Autodesk Inventor part; units mm, degrees
ref_plane "Work Plane2" through (-342.433406, -360.707407, -533) normal (0, 0, -1) x (0, 1, 0)
ref_plane "YZ Plane" through (0, 0, 0) normal (1, 0, 0) x (0, 1, 0)
ref_plane "XZ Plane" through (0, 0, 0) normal (0, 1, 0) x (-1, 0, 0)
ref_plane "Work Plane1" through (0, 0, 0) normal (0, 0, 1) x (1, 0, 0)
sketch "Sketch1" plane through (0, 0, 0) normal (0, 0, 1) x (1, 0, 0)
  arc A0 (173.074137, -21.982113) -> (67.5, 160.877656) centre (67.5, 38.971143) ccw
  line L0 (67.5, 160.877656) -> (23, 160.877656)
  line L1 (150.824137, -60.520244) -> (173.074137, -21.982113)
  line L2 (23, 162.377656) -> (67.5, 162.377656)
  arc A1 (174.373175, -22.732113) -> (67.5, 162.377656) centre (67.5, 38.971143) ccw
  line L3 (174.373175, -22.732113) -> (152.123175, -61.270244)
  line L4 (150.824137, -60.520244) -> (152.123175, -61.270244)
  line L5 (23, 160.877656) -> (23, 162.377656)
  point P0 (0, 0)
  dimension "d0" = 1.5
ref_plane "Work Plane2" through (-342.433406, -360.707407, -533) normal (0, 0, -1) x (0, 1, 0)
extrude "Extrusion1" add sketch "Sketch1" against normal blind 551
sketch "Sketch2" plane through (0, 0, 0) normal (0, 0, 1) x (1, 0, 0)
  line L0 (174.373175, -22.732113) -> (152.123175, -61.270244)
  arc A0 (174.373175, -22.732113) -> (67.5, 162.377656) centre (67.5, 38.971143) ccw
  line L1 (23, 162.377656) -> (67.5, 162.377656)
  line L2 (23, 162.377656) -> (67.5, 162.377656)
  line L3 (67.5, 162.377656) -> (67.5, 147.377656)
  line L4 (67.5, 147.377656) -> (23, 147.377656)
  line L5 (23, 147.377656) -> (23, 162.377656)
  line L6 (152.123175, -61.270244) -> (174.373175, -22.732113)
  line L7 (174.373175, -22.732113) -> (161.382794, -15.232113)
  line L8 (161.382794, -15.232113) -> (139.132794, -53.770244)
  line L9 (139.132794, -53.770244) -> (152.123175, -61.270244)
  point P0 (0, 0)
  dimension "d3" = 15
  dimension "d4" = 15
extrude "Extrusion2" add sketch "Sketch2" along normal blind 1.5
fillet "Fillet4" radius 6 4 edges at (161.3828, -15.2321, 0.75) (139.1328, -53.7702, 0.75) (23, 147.3777, 0.75) (67.5, 147.3777, 0.75)
sketch "Sketch5" plane through (0, 0, 1.5) normal (0, 0, 1) x (1, 0, 0)
  arc A0 (61.5, 147.377656) -> (67.5, 153.377656) centre (61.5, 153.377656) ccw
  arc A1 (23, 153.377656) -> (29, 147.377656) centre (29, 153.377656) ccw
  arc A2 (142.132794, -48.574091) -> (144.328946, -56.770244) centre (147.328946, -51.574091) ccw
  line L0 (144.328946, -56.770244) -> (152.123175, -61.270244)
  line L1 (174.373175, -22.732113) -> (166.578946, -18.232113)
  arc A3 (166.578946, -18.232113) -> (158.382794, -20.428266) centre (163.578946, -23.428266) ccw
  line L2 (158.382794, -20.428266) -> (142.132794, -48.574091)
  circle A4 centre (29, 153.377656) radius 2
  circle A5 centre (61.5, 153.377656) radius 2
  circle A6 centre (163.578946, -23.428266) radius 2
  circle A7 centre (147.328946, -51.574091) radius 2
  line L3 (152.123175, -61.270244) -> (174.373175, -22.732113)
  point P0 (0, 0)
  dimension "d17" = 4
  dimension "d18" = 4
  dimension "d19" = 4
  dimension "d20" = 4
extrude "Extrusion5" cut sketch "Sketch5" against normal blind 2 contours A4 | A5 | A6 | A7
fillet "Fillet5" radius 1.5 2 edges at (45.25, 160.8777, 0) (161.9491, -41.2512, 0)
ref_plane "Work Plane5" through (0, 0, -275.5) normal (0, 0, 1) x (1, 0, 0)
mirror "Mirror3" about plane through (0, 0, -275.5) normal (0, 0, 1) of "Extrusion2", "Extrusion5", "Fillet4", "Fillet5"
sketch "Sketch7" plane through (0, 0, -551) normal (0, 0, -1) x (-1, 0, 0)
  line L0 (-67.5, 160.877656) -> (-67.5, 162.377656)
  arc A0 (-67.5, 162.377656) -> (-174.373175, -22.732113) centre (-67.5, 38.971143) ccw
  line L1 (-174.373175, -22.732113) -> (-173.074137, -21.982113)
  arc A1 (-67.5, 160.877656) -> (-173.074137, -21.982113) centre (-67.5, 38.971143) ccw
  point P0 (0, 0)
extrude "Extrusion7" cut sketch "Sketch7" against normal blind 2
sketch "Sketch8" plane through (0, 0, 0) normal (0, 0, 1) x (1, 0, 0)
  line L0 (67.5, 162.377656) -> (67.5, 160.877656)
  arc A0 (173.074137, -21.982113) -> (67.5, 160.877656) centre (67.5, 38.971143) ccw
  line L1 (173.074137, -21.982113) -> (174.373175, -22.732113)
  arc A1 (174.373175, -22.732113) -> (67.5, 162.377656) centre (67.5, 38.971143) ccw
  point P0 (0, 0)
extrude "Extrusion8" cut sketch "Sketch8" against normal blind 2
fillet "Fillet7" radius 3 4 edges at (45.25, 162.3777, 1.5) (163.2482, -42.0012, 1.5) (163.2482, -42.0012, -552.5) (45.25, 162.3777, -552.5)
properties material "Aluminum 6061"
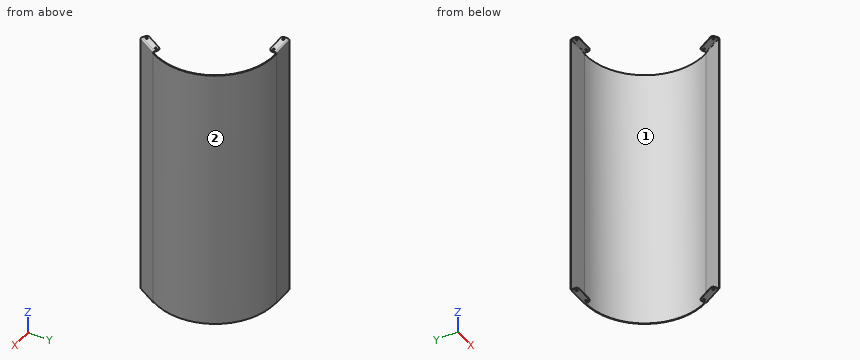
Check sheet for the modelled part. Datum: model origin and axes. Units: mm. Face numbers are marked on the shaded views. Round coordinates to 2 decimals unless told otherwise and drop trailing zeros. Loops run counter-clockwise (first coordinate to the right, second up) from the corner with the lowest first, then second, coordinate; pieces in that order, holes last. Notation, with made-up numbers: M -36,-4 L -20,-4 A13 cw -20,17 Z; hole C -4,28 d7. An arc over 180 degrees is marked long. One line per item, written item: value.
(1) Sectioned sample at C-C, the plane x = 85.5. Record the cut outline in (y, z).
Computed values:
outline: M 159.54,-549 L 161.06,-549 L 161.06,-2 L 159.54,-2 Z
(2) Sectioned sample at A-A, the plane x = 180.5. Record the cut outline in (y, z).
Computed values:
outline: M -10.63,-549 L -6.77,-549 L -6.77,-2 L -10.63,-2 Z; M 84.71,-549 L 88.57,-549 L 88.57,-2 L 84.71,-2 Z
(3) Release check for a two-part mould opening along Y. For the marked faces 1 and 2 record: +Y half, -Y half, draft (parallel to the pull), parting line (faces both ways), or undercut.
Computed values:
face 1: undercut
face 2: parting line
(4) Sectioned sample at B-B, the plane z = -455. Record the cut outline in (x, y), then the cut area to 3 significant figures.
Computed values:
outline: M 23,160.88 L 67.5,160.88 A121.91 cw 173.07,-21.98 L 150.82,-60.52 L 152.12,-61.27 L 174.37,-22.73 A123.41 ccw 67.5,162.38 L 23,162.38 Z
area: 519 mm^2
(5) Sectioned sample at D-D, the plane x = 121.5. Record the cut outline in (y, z).
Computed values:
outline: M 148.27,-549 L 149.94,-549 L 149.94,-2 L 148.27,-2 Z
(6) Thickness scan on line 1 (X direction, y = 42.5, z = -138); line 2 (Y direction, x = 156, z = -414.5); line 3 (Y direction, x = 53.5, z = -440). Record the ranges inside material, lowest first.
Computed values:
line 1: x = 189.36 to 190.86
line 2: y = -54.56 to -51.56, 122.81 to 124.98
line 3: y = 160.88 to 162.38
(7) Depth check by flat-ended pin: pin 1 Ø1.5 at (y, z) = (30.5, -110) entering from -X; pin 2 Ø6.5 at (x, y) = (61.5, 153.38) entering from +Z; pin 3 Ø8 at (y, z) = (-37, -59) entering from +X (3 decimals); pin 4 Ø1.5 at (x, z) = (133.5, -340) entering from -Y. Enter the tip coordinate at first touch or a pass-through.
Computed values:
pin 1: stops at x = 189.06
pin 2: stops at z = 1.5
pin 3: stops at x = 168.445
pin 4: stops at y = 140.98
